Part model, mm, in its own coordinate system. Face numbers are marked on the shaded views. A direction names the side the tool comes from. Round coordinates to 2 decimals unless told otherwise and drop trailing zeros. Write each loop counter-clockwise with the first axis right and the second up, starting at its lowest first coordinate (ties: lowest second). Pieces come first, ordered by that corner, then holes. Notation, with made-up numbers: M -9,75 L 5,75 A24 ccw 5,88 Z; hole C 48,24.25 d3. An arc over 180 degrees is marked long. One line per question, with ' | ' between items. Start each with the question number.
1) Wall check: probe 1 along X at (y, z) = (1.9, 2.6); probe 2 along Y at (x, z) = (0, 68.05); probe 3 along X at (y, z) = (-5.5, 67.5). Give the ranges that are in metal, low to high. Write a range as [from, to].
2) Saw through at B-B (z = -2.6). List the corners of the cut face in (x, y).
3) Drop flat-ended pins along their axis: pin 1 Ø5 at (x, z) = (3.5, -13) entering from +Y; pin 2 Ø3 at (x, z) = (-13.4, -29.4) entering from -Y; pin 3 Ø1.3 at (x, z) = (-9, 66.5) entering from +Y. Give the stop position or say it passes through.
4) Saw through at A-A (z = -44). List the corners of the cut face in (x, y).
5) Saw through at C-C (x = 0). Give the number of separate pieces and of enclosed holes in the cut face, plus the area to 3 significant figures.
6) Tool access for the marked faces 1, 2 and 3: list every direction of +Z, -Z, +X, -X, +Y, -Y with a clear straight run to the whole face (end or side of a thin tool).
7) Saw through at D-D (z = 61.4). List the corners of the cut face in (x, y), plus the area to 3 significant figures.
```python
from build123d import *

# Parameters (mm, degrees)
SKETCH1_W               = 32
SKETCH1_H               = 128
BOSS_EXTRUDE1_DEPTH     = 4
SKETCH4_R               = 1.25
CUT_EXTRUDE2_DEPTH      = 10
SKETCH5_R               = 1.25
CUT_EXTRUDE3_DEPTH      = 10
CUT_EXTRUDE4_DEPTH      = 1.65
LPATTERN3_COUNT         = 4
LPATTERN3_PITCH         = 32
CUT_EXTRUDE5_DEPTH      = 1.65
LPATTERN4_COUNT         = 4
LPATTERN4_PITCH         = 32
SKETCH8_W               = 24.3
SKETCH8_H               = 24.3
CUT_EXTRUDE6_DEPTH      = 10
BOSS_EXTRUDE2_DEPTH     = 4.5
SKETCH11_W              = 10.2
SKETCH11_H              = 71.7
CUT_EXTRUDE7_DEPTH      = 72.92530848
CUT_EXTRUDE8_DEPTH      = 3
SKETCH12_R              = 2.25
CUT_EXTRUDE9_DEPTH      = 3
MIRROR3_COPY_1_DEPTH    = 3
MIRROR3_COPY_2_SKETCH_R = 2.25
MIRROR3_COPY_2_DEPTH    = 3


with BuildPart() as part:
    # Sketch1 → Boss-Extrude1 (new body)
    with BuildSketch(Plane(origin=(0, 0, 0), x_dir=(1, 0, 0), z_dir=(0, 1, 0))):
        Rectangle(SKETCH1_W, SKETCH1_H)
    extrude(amount=BOSS_EXTRUDE1_DEPTH)

    # Sketch4 → Cut-Extrude2 (cut)
    with BuildSketch(Plane.XZ):
        with Locations(Location((13.4, 61.4, 0), (0, 0, 270))):
            Circle(SKETCH4_R)
    cut_extrude2 = extrude(amount=-CUT_EXTRUDE2_DEPTH, mode=Mode.SUBTRACT)

    # Sketch5 → Cut-Extrude3 (cut)
    with BuildSketch(Plane.XZ):
        with Locations(Location((-13.4, -61.4, 0), (0, 0, 270))):
            Circle(SKETCH5_R)
    cut_extrude3 = extrude(amount=-CUT_EXTRUDE3_DEPTH, mode=Mode.SUBTRACT)

    # Sketch6 → Cut-Extrude4 (cut)
    with BuildSketch(Plane(origin=(0, 4, 0), x_dir=(1, 0, 0), z_dir=(0, 1, 0))):
        Polygon((-15.400518683, 62.555), (-13.4, 63.71), (-11.399481317, 62.555), (-11.399481317, 60.245), (-13.4, 59.09), (-15.400518683, 60.245), align=None)
    cut_extrude4 = extrude(amount=-CUT_EXTRUDE4_DEPTH, mode=Mode.SUBTRACT)

    # LPattern3: Cut-Extrude3, Cut-Extrude4 ×4
    with Locations(*[(0, 0, i * LPATTERN3_PITCH) for i in range(1, LPATTERN3_COUNT)]):
        add(cut_extrude3, mode=Mode.SUBTRACT)
        add(cut_extrude4, mode=Mode.SUBTRACT)

    # Sketch7 → Cut-Extrude5 (cut)
    with BuildSketch(Plane(origin=(0, 4, 0), x_dir=(1, 0, 0), z_dir=(0, 1, 0))):
        Polygon((13.4, -59.09), (11.399481317, -60.245), (11.399481317, -62.555), (13.4, -63.71), (15.400518683, -62.555), (15.400518683, -60.245), align=None)
    cut_extrude5 = extrude(amount=-CUT_EXTRUDE5_DEPTH, mode=Mode.SUBTRACT)

    # LPattern4: Cut-Extrude2, Cut-Extrude5 ×4
    with Locations(*[(0, 0, -i * LPATTERN4_PITCH) for i in range(1, LPATTERN4_COUNT)]):
        add(cut_extrude2, mode=Mode.SUBTRACT)
        add(cut_extrude5, mode=Mode.SUBTRACT)

    # Sketch8 → Cut-Extrude6 (cut)
    with BuildSketch(Plane.XZ):
        with Locations((0, 48)):
            Rectangle(SKETCH8_W, SKETCH8_H)
    cut_extrude6 = extrude(amount=-CUT_EXTRUDE6_DEPTH, mode=Mode.SUBTRACT)

    # Mirror1: Cut-Extrude6 across plane
    add(cut_extrude6.mirror(Plane.XY), mode=Mode.SUBTRACT)

    # Sketch9 → Boss-Extrude2 (add)
    with BuildSketch(Plane(origin=(0, 0, -64), x_dir=(-1, 0, 0), z_dir=(0, 0, -1))):
        Polygon((-16, 12), (-5, 12), (-5, 15), (5, 15), (5, 12), (16, 12), (16, -8), (5, -8), (5, -11), (-5, -11), (-5, -8), (-16, -8), align=None)
    boss_extrude2 = extrude(amount=BOSS_EXTRUDE2_DEPTH)

    # Sketch11 → Cut-Extrude7 (cut, through all)
    with BuildSketch(Plane.XZ):
        Rectangle(SKETCH11_W, SKETCH11_H)
    extrude(amount=-CUT_EXTRUDE7_DEPTH, mode=Mode.SUBTRACT)

    # Sketch10 → Cut-Extrude8 (cut)
    with BuildSketch(Plane.XY.offset(-64)):
        Polygon((-2.52, 13.864768035), (2.52, 13.864768035), (5.04, 9.5), (2.52, 5.135231965), (-2.52, 5.135231965), (-5.04, 9.5), align=None)
    cut_extrude8 = extrude(amount=-CUT_EXTRUDE8_DEPTH, mode=Mode.SUBTRACT)

    # Sketch12 → Cut-Extrude9 (cut)
    with BuildSketch(Plane.XY.offset(-67)):
        with Locations((0, 9.5)):
            Circle(SKETCH12_R)
    cut_extrude9 = extrude(amount=-CUT_EXTRUDE9_DEPTH, mode=Mode.SUBTRACT)

    # Mirror2: Cut-Extrude8, Cut-Extrude9 across plane
    add(cut_extrude8.mirror(Plane.ZX.offset(2)), mode=Mode.SUBTRACT)
    add(cut_extrude9.mirror(Plane.ZX.offset(2)), mode=Mode.SUBTRACT)

    # Mirror3: Boss-Extrude2, Cut-Extrude8, Cut-Extrude9 across plane
    add(boss_extrude2.mirror(Plane.XY))
    add(cut_extrude8.mirror(Plane.XY), mode=Mode.SUBTRACT)
    add(cut_extrude9.mirror(Plane.XY), mode=Mode.SUBTRACT)

    # Mirror3 copy 1 sketch → Mirror3 copy 1 (cut)
    with BuildSketch(Plane(origin=(0, 4, 64), x_dir=(1, 0, 0), z_dir=(0, 0, -1))):
        Polygon((-2.52, 13.864768035), (2.52, 13.864768035), (5.04, 9.5), (2.52, 5.135231965), (-2.52, 5.135231965), (-5.04, 9.5), align=None)
    extrude(amount=-MIRROR3_COPY_1_DEPTH, mode=Mode.SUBTRACT)

    # Mirror3 copy 2 sketch → Mirror3 copy 2 (cut)
    with BuildSketch(Plane(origin=(0, 4, 67), x_dir=(1, 0, 0), z_dir=(0, 0, -1))):
        with Locations((0, 9.5)):
            Circle(MIRROR3_COPY_2_SKETCH_R)
    extrude(amount=-MIRROR3_COPY_2_DEPTH, mode=Mode.SUBTRACT)


solid = part.part
```
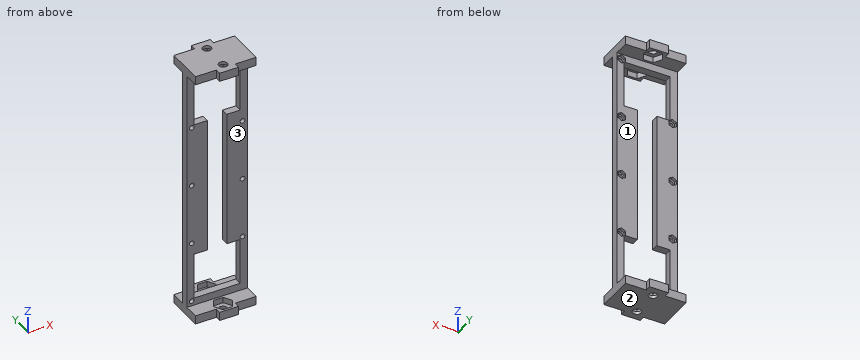
Answer key:
1) probe 1: x = [-16, -14.65], [-12.15, -5.1], [5.1, 16] | probe 2: y = [-11, -7.75], [-3.25, 7.25], [11.75, 15] | probe 3: x = [-16, -2.25], [2.25, 16]
2) outline: M -16,0 L -5.1,0 L -5.1,4 L -16,4 Z; M 5.1,0 L 12.15,0 L 12.15,2.35 L 11.4,2.35 L 11.4,4 L 5.1,4 Z; M 14.65,0 L 16,0 L 16,4 L 15.4,4 L 15.4,2.35 L 14.65,2.35 Z
3) pin 1: stops at y = 4 | pin 2: stops at y = 0 | pin 3: stops at y = 12
4) outline: M -16,0 L -12.15,0 L -12.15,4 L -16,4 Z; M 12.15,0 L 16,0 L 16,4 L 12.15,4 Z
5) separate pieces: 6 | enclosed holes: 0 | area: 133 mm2
6) face 1: +X, -X, +Y | face 2: -Z, +X, -X, +Y, -Y | face 3: +X, -X, -Y
7) outline: M -16,0 L 12.15,0 L 12.15,2.35 L 11.4,2.35 L 11.4,4 L -16,4 Z; M 14.65,0 L 16,0 L 16,4 L 15.4,4 L 15.4,2.35 L 14.65,2.35 Z | area: 116 mm2
